from build123d import *

# Parameters (mm, degrees)
F0_W         = 168
F0_H         = 36
F1_DEPTH     = 14
F3_DEPTH     = 36.001
F5_DEPTH     = 41
F6_R         = 5.25
F7_DEPTH     = 55.001
F8_W         = 20
F8_H         = 20
F9_DEPTH     = 6.5
F10_W        = 67
F10_H        = 20
F11_DEPTH    = 2
F12_T1_DEPTH = 34.1421356237
F14_DEPTH    = 25
F16_DEPTH    = 36.001


# Not quite as in the source:
# - a fillet or chamfer that OpenCascade refuses, or shapes differently, is made with other operations: its cross-section is extruded or revolved along the edge and cut away or added


with BuildPart() as f1:
    # F0 (on Front) → F1 (new body)
    with BuildSketch(Plane.XZ):
        Rectangle(F0_W, F0_H)
    extrude(amount=F1_DEPTH)

    # F2 (on face) → F3 (cut, through all)
    with BuildSketch(Plane(origin=(0, 0, -18), x_dir=(1, 0, 0), z_dir=(0, 0, -1))):
        Polygon((-84, 14), (-84, 0), (-80, 14), align=None)
        Polygon((80, 14), (84, 0), (84, 14), align=None)
    extrude(amount=-F3_DEPTH, mode=Mode.SUBTRACT)

    # F4 (on face) → F5 (join)
    with BuildSketch(Plane.XZ.offset(14)):
        with BuildLine():
            ThreePointArc((39.0512483795, -18), (43, 0), (39.0512483795, 18))
            Line((39.0512483795, 18), (-39.0512483795, 18))
            ThreePointArc((-39.0512483795, 18), (-43, 0), (-39.0512483795, -18))
            Line((-39.0512483795, -18), (39.0512483795, -18))
        make_face()
    extrude(amount=F5_DEPTH)

    # F6 (on face) → F7 (cut, through all)
    with BuildSketch(Plane.XZ.offset(55)):
        with Locations((36.25, 0)):
            Circle(F6_R)
        with Locations((-31, 0)):
            Circle(F6_R)
    extrude(amount=-F7_DEPTH, mode=Mode.SUBTRACT)

    # F8 (on face) → F9 (cut)
    with BuildSketch(Plane(origin=(0, 0, 0), x_dir=(-1, 0, 0), z_dir=(0, 1, 0))):
        with Locations((-36.25, 0)):
            Rectangle(F8_W, F8_H)
        with Locations((31, 0)):
            Rectangle(F8_W, F8_H)
    extrude(amount=-F9_DEPTH, mode=Mode.SUBTRACT)

    # F10 (on face) → F11 (cut)
    with BuildSketch(Plane(origin=(0, 0, 0), x_dir=(-1, 0, 0), z_dir=(0, 1, 0))):
        with Locations((41.5, 0)):
            Rectangle(F10_W, F10_H)
        with Locations((-41.5, 0)):
            Rectangle(F10_W, F10_H)
    extrude(amount=-F11_DEPTH, mode=Mode.SUBTRACT)

    # F12: fillet of radius 3 on 4 edges, made by hand

    # F12_s2 → F12_t1 (join)
    with BuildSketch(Plane.XY.offset(-17.0710678119)):
        with BuildLine():
            ThreePointArc((72.1715728753, -2), (73.9036236828, -1.4494897428), (75, 0))
            Line((75, 0), (75, -2))
            Line((75, -2), (72.1715728753, -2))
        make_face()
        with BuildLine():
            ThreePointArc((10.8284271247, -2), (9.0963763172, -1.4494897428), (8, 0))
            Line((8, 0), (8, -2))
            Line((8, -2), (10.8284271247, -2))
        make_face()
        with BuildLine():
            ThreePointArc((-72.1715728753, -2), (-73.9036236828, -1.4494897428), (-75, 0))
            Line((-75, 0), (-75, -2))
            Line((-75, -2), (-72.1715728753, -2))
        make_face()
        with BuildLine():
            ThreePointArc((-10.8284271247, -2), (-9.0963763172, -1.4494897428), (-8, 0))
            Line((-8, 0), (-8, -2))
            Line((-8, -2), (-10.8284271247, -2))
        make_face()
    extrude(amount=F12_T1_DEPTH)

    # F13 (on face) → F14 (cut)
    with BuildSketch(Plane.XZ.offset(14)):
        with BuildLine():
            ThreePointArc((-67.6350200021, 5), (-72.6350200021, 0), (-67.6350200021, -5))
            Line((-67.6350200021, -5), (-59.6350200021, -5))
            ThreePointArc((-59.6350200021, -5), (-54.6350200021, 0), (-59.6350200021, 5))
            Line((-59.6350200021, 5), (-67.6350200021, 5))
        make_face()
        with BuildLine():
            ThreePointArc((54.5760053992, 0), (56.0404714933, -3.5355339059), (59.5760053992, -5))
            Line((59.5760053992, -5), (67.5760053992, -5))
            ThreePointArc((67.5760053992, -5), (71.1115393052, -3.5355339059), (72.5760053992, 0))
            ThreePointArc((72.5760053992, 0), (71.1115393052, 3.5355339059), (67.5760053992, 5))
            Line((67.5760053992, 5), (59.5760053992, 5))
            ThreePointArc((59.5760053992, 5), (56.0404714933, 3.5355339059), (54.5760053992, 0))
        make_face()
    extrude(amount=-F14_DEPTH, mode=Mode.SUBTRACT)

    # F15 (on face) → F16 (cut, through all)
    with BuildSketch(Plane.XY.offset(18)):
        with BuildLine():
            Line((22, -43), (19, -43))
            ThreePointArc((19, -43), (0, -24), (-19, -43))
            Line((-19, -43), (-22, -43))
            Line((-22, -43), (-22, -55))
            Line((-22, -55), (0, -55))
            Line((0, -55), (22, -55))
            Line((22, -55), (22, -43))
        make_face()
    extrude(amount=-F16_DEPTH, mode=Mode.SUBTRACT)


solid = f1.part
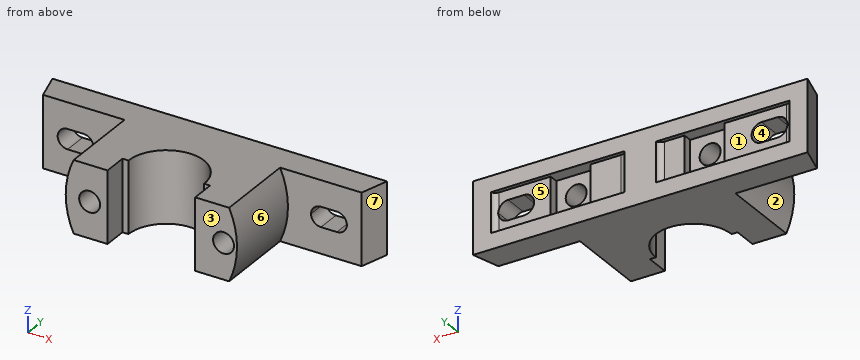
Design review of the part built by this model. Coordinates are the model's own, in mm. Face numbers are marked on the shaded views. A direction names the side the tool comes from. Coordinates: 2 decimals unless noted, no trailing zeros. Write each loop counter-clockwise with the first axis right and the second up, starting at its lowest first coordinate (ties: lowest second). Pieces come first, ordered by that corner, then holes. Notation, with made-up numbers: (35.5, -20) -> (64.5, -20) arc R9 ccw to (64.5, -10) -> close; hole circle Ø11 at (25, 65.25). An arc over 180 degrees is marked (long way). Write each question's results on one line, items separated by ' | '. Start each with the question number.
(1) Tool access review of the marked faces 4, 5, 6 and 7: name each direction out of +Z, -Z, +X, -X, +Y, -Y from which nothing blocks a thin tool from reaching the whole face with its end or side.
(2) Take a section at A-A on y = -37.5. Write out the cut boundary in (x, z).
(3) Take a section at B-B on x = -31. Write out the cut boundary in (y, z).
(4) The part is to be moulded in two halves that separate along Z. For the marked faces 1, 2 and 3, say which applies: pulls with the +Z half, pulls with the -Z half, needs draft (parallel to the pull), parting line crosses it, or undercut.
(5) For line 1 along Z through (x, y) = (-31, -44); line 2 along Z through (x, y) = (-28, -2.5); line 3 along X through (y, z) = (-40.5, 1.5), list the stretches that pass through material, from the lowest coordinate up. Write a range as from..to.
(6) Take a section at C-C on z = -12.5. Write out the cut boundary in (x, y), and give its area (3 significant figures).
(7) Take a section at D-D on y = -16. Write out the cut boundary in (x, z).
(8) Clearance check with flat-ended pins moving along their axes: P1, Ø1.3, axis at y = -3.5, z = -2.5, coming from the -X side; P2, Ø1.5, axis at y = -32.5, z = -11.5, coming from the +X side; P3, Ø5, axis at y = -4.5, z = -5, coming from the +X side. State where each tip first meets the part, or that it passes through.
Results found:
1) face 4: +Y, -Y | face 5: +Y | face 6: +X, -Y | face 7: +Z, -Z, +X, -Y
2) outline: (-39.05, -18) -> (-18.19, -18) -> (-18.19, 18) -> (-39.05, 18) arc R43 ccw to start; (18.19, -18) -> (39.05, -18) arc R43 ccw to (39.05, 18) -> (18.19, 18) -> close; hole circle Ø10.5 at (-31, 0); hole circle Ø10.5 at (36.25, 0)
3) outline: (-55, -18) -> (0, -18) -> (0, -10) -> (-6.5, -10) -> (-6.5, -5.25) -> (-55, -5.25) -> close; (-55, 5.25) -> (-6.5, 5.25) -> (-6.5, 10) -> (0, 10) -> (0, 18) -> (-55, 18) -> close
4) face 1: undercut | face 2: parting line crosses it | face 3: needs draft
5) line 1: z = -18..-5.25, 5.25..18 | line 2: z = -18..-10, 10..18 | line 3: x = -42.97..-36.03, -25.97..-18.83, 18.83..31.22, 41.28..42.97
6) outline: (-84, 0) -> (-80, -14) -> (-41.14, -14) -> (-41.14, -55) -> (-22, -55) -> (-22, -43) -> (-19, -43) arc R19 cw to (19, -43) -> (22, -43) -> (22, -55) -> (41.14, -55) -> (41.14, -14) -> (80, -14) -> (84, 0) -> close | area: 4,570 mm2
7) outline: (-39.05, -18) -> (39.05, -18) arc R43 ccw to (39.05, 18) -> (-39.05, 18) arc R43 ccw to start; hole circle Ø10.5 at (-31, 0); hole circle Ø10.5 at (36.25, 0)
8) P1: stops at x = -83.19 | P2: stops at x = 41.63 | P3: stops at x = 83.43
